from build123d import *

# Parameters (mm, degrees)
BOSS_EXTRUDE2_DEPTH = 21
SKETCH2_W           = 12
SKETCH2_H           = 4.5
BOSS_EXTRUDE3_DEPTH = 15


with BuildPart() as part:
    # Sketch1 → Boss-Extrude2 (new body)
    with BuildSketch(Plane.XY):
        Polygon((1, 2), (1, 10), (-1.5, 10), (-1.5, 2), (-13, 2), (-13, -2), (13, -2), (13, 2), align=None)
    extrude(amount=BOSS_EXTRUDE2_DEPTH)

    # Sketch2 → Boss-Extrude3 (add)
    with BuildSketch(Plane.ZY.offset(13)):
        with Locations((10.5, 1.75)):
            Rectangle(SKETCH2_W, SKETCH2_H)
    extrude(amount=BOSS_EXTRUDE3_DEPTH)


solid = part.part
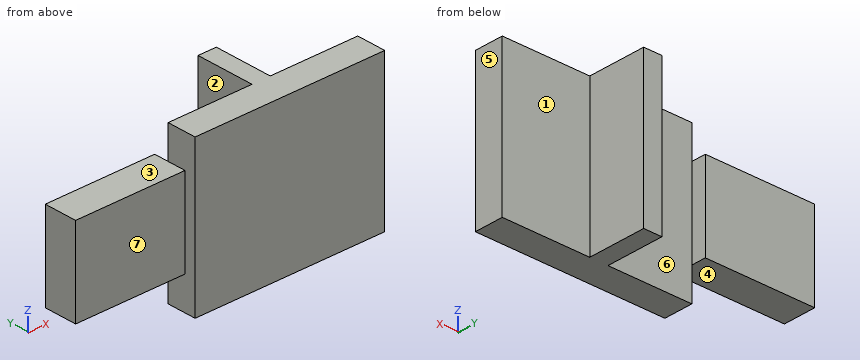
Source: CAD feature listing. Evaluate the final solid. Frame: model axes, mm. Face numbers are marked on the shaded views. A direction names the side the tool comes from. Coordinates: 2 decimals unless noted, no trailing zeros. Write each loop counter-clockwise with the first axis right and the second up, starting at its lowest first coordinate (ties: lowest second). Pieces come first, ordered by that corner, then holes. Notation, with made-up numbers: M -20.75,-2 L 13.25,-2 A7 cw 13.25,3 Z; hole C -11.75,-14 d5. An arc over 180 degrees is marked long. Use a Markdown table: item, result.
1) First-contact query: pin 1 Ø6 at (x, z) = (-9, 8.5) entering from +Y; pin 2 Ø6 at (y, z) = (5, 3) entering from -X; pin 3 Ø2.5 at (y, z) = (4, 12) entering from +X; pin 4 Ø5 at (x, y) = (-22, 0.5) entering from -Z. Flat tips, straight axial feed; report the tip coordinate or a pass-through.
Conclusion:
| item | result |
|---|---|
| pin 1 | stops at y = 2 |
| pin 2 | stops at x = -28 |
| pin 3 | stops at x = 1 |
| pin 4 | stops at z = 4.5 |
2) Section A-A, the plane y = 0.75. Output: boundary loops of the cut face in (x, z).
Conclusion:
| item | result |
|---|---|
| outline | M -28,4.5 L -13,4.5 L -13,0 L 13,0 L 13,21 L -13,21 L -13,16.5 L -28,16.5 Z |
3) Section B-B, the plane z = 18.5. Output: boundary loops of the cut face in (x, y), then the cut area to 3 significant figures.
Conclusion:
| item | result |
|---|---|
| outline | M -13,-2 L 13,-2 L 13,2 L 1,2 L 1,10 L -1.5,10 L -1.5,2 L -13,2 Z |
| area | 124 mm^2 |
4) Section C-C, the plane x = -12. Output: boundary loops of the cut face in (y, z).
Conclusion:
| item | result |
|---|---|
| outline | M -2,0 L 2,0 L 2,21 L -2,21 Z |
5) Mould query, pull axis X, two halves, no side actions, for the marked faces 5, 6 and 7. Classes: pulls with the +X half, pulls with the -X half, needs draft (parallel to the pull), parting line crosses it, or undercut.
Conclusion:
| item | result |
|---|---|
| face 5 | pulls with the +X half |
| face 6 | undercut |
| face 7 | needs draft |
6) Reachability of the marked faces 1, 2, 3 and 4 from +Z, -Z, +X, -X, +Y, -Y: full face, straight path, thin tool, end or side. Return the list, or none.
Conclusion:
| item | result |
|---|---|
| face 1 | +Z, -Z, +X, +Y |
| face 2 | +Z, -Z, +Y |
| face 3 | +Z, -X, +Y, -Y |
| face 4 | -Z, -X, +Y, -Y |
7) Ray query, L1, parallel to X at y = 2.75, z = 5.5; L2, parallel to Y at x = 8, z = 20; L3, parallel to X at y = 9, z = 2. Return the intervals inside material, ascending.
Conclusion:
| item | result |
|---|---|
| L1 | x = -28 to -13, -1.5 to 1 |
| L2 | y = -2 to 2 |
| L3 | x = -1.5 to 1 |
8) Section D-D, the plane z = 11.5. Output: boundary loops of the cut face in (x, y), then the cut area to 4 significant figures.
Conclusion:
| item | result |
|---|---|
| outline | M -28,-0.5 L -13,-0.5 L -13,-2 L 13,-2 L 13,2 L 1,2 L 1,10 L -1.5,10 L -1.5,2 L -13,2 L -13,4 L -28,4 Z |
| area | 191.5 mm^2 |
